Can you work these out from the model? Positions are in its coordinate system, mm. Give positions to 0.01 mm unless a question says otherwise; leave off trailing zeros. Write each loop counter-clockwise with the first axis right and the second up, starting at its lowest first coordinate (ties: lowest second). Pieces come first, ordered by that corner, then holes.
1. If I drill on probe 1 along Y at (x, z) = (-19.05, 1.2) (3 decimals); probe 2 along X at (y, z) = (-1, 0.4); probe 3 along Y at (x, z) = (0, 0.9) (3 decimals), over which ranges is the centre line in solid material (lowest first)?
2. Suppose I cut it at C-C (x = 0). Please give me the cut outline in (y, z) (1 decimal), and give its area (3 significant figures).
3. Suppose I cut it at A-A (z = 0.45). Please give me the cut outline in (x, y) (3 decimals), and give its area (3 significant figures).
4. Suppose I cut it at B-B (y = 0). Please give me the cut outline in (x, z), and give its area (3 significant figures).
5. Suppose I cut it at D-D (y = -6). Please give me the cut outline in (x, z).
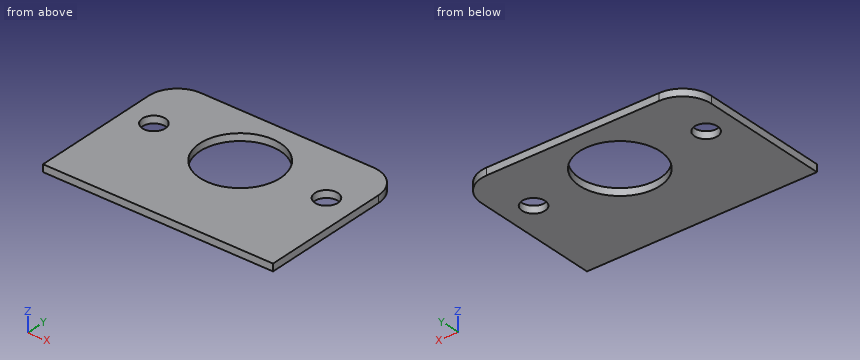
```python
from build123d import *

# Parameters (mm, degrees)
SKETCH1_W           = 50.8
SKETCH1_H           = 25.4
SKETCH1_R           = 8.89
SKETCH1_R_2         = 2.54
BOSS_EXTRUDE1_DEPTH = 1.5875
SKETCH3_W           = 50.8
SKETCH3_H           = 9.525
BOSS_EXTRUDE2_DEPTH = 1.5875
FILLET1_R           = 6.35


with BuildPart() as part:
    # Sketch1 → Boss-Extrude1 (new body)
    with BuildSketch(Plane.XY):
        Rectangle(SKETCH1_W, SKETCH1_H)
        Circle(SKETCH1_R, mode=Mode.SUBTRACT)
        with Locations((19.05, 0)):
            Circle(SKETCH1_R_2, mode=Mode.SUBTRACT)
        with Locations((-19.05, 0)):
            Circle(SKETCH1_R_2, mode=Mode.SUBTRACT)
    extrude(amount=BOSS_EXTRUDE1_DEPTH)

    # Sketch3 → Boss-Extrude2 (add)
    with BuildSketch(Plane.XY):
        with Locations((0, -17.4625)):
            Rectangle(SKETCH3_W, SKETCH3_H)
    extrude(amount=BOSS_EXTRUDE2_DEPTH)

    # Fillet1
    fillet1_edges = [part.edges().sort_by_distance(p)[0] for p in [
        (-25.4, 12.7, 0.79375),
        (25.4, 12.7, 0.79375),
    ]]
    fillet(fillet1_edges, radius=FILLET1_R)


solid = part.part
```
Checks:
1. probe 1: y = -22.225 to -2.54, 2.54 to 12.7
1. probe 2: x = -25.4 to -21.38, -16.72 to -8.83, 8.83 to 16.72, 21.38 to 25.4
1. probe 3: y = -22.225 to -8.89, 8.89 to 12.7
2. outline: (-22.2, 0) - (-8.9, 0) - (-8.9, 1.6) - (-22.2, 1.6) - close; (8.9, 0) - (12.7, 0) - (12.7, 1.6) - (8.9, 1.6) - close
2. area: 27.2 mm2
3. outline: (-25.4, -22.225) - (25.4, -22.225) - (25.4, 6.35) arc R6.35 ccw to (19.05, 12.7) - (-19.05, 12.7) arc R6.35 ccw to (-25.4, 6.35) - close; hole circle Ø5.08 at (-19.05, 0); hole circle Ø17.78 at (0, 0); hole circle Ø5.08 at (19.05, 0)
3. area: 1,470 mm2
4. outline: (-25.4, 0) - (-21.59, 0) - (-21.59, 1.59) - (-25.4, 1.59) - close; (-16.51, 0) - (-8.89, 0) - (-8.89, 1.59) - (-16.51, 1.59) - close; (8.89, 0) - (16.51, 0) - (16.51, 1.59) - (8.89, 1.59) - close; (21.59, 0) - (25.4, 0) - (25.4, 1.59) - (21.59, 1.59) - close
4. area: 36.3 mm2
5. outline: (-25.4, 0) - (-6.56, 0) - (-6.56, 1.59) - (-25.4, 1.59) - close; (6.56, 0) - (25.4, 0) - (25.4, 1.59) - (6.56, 1.59) - close
